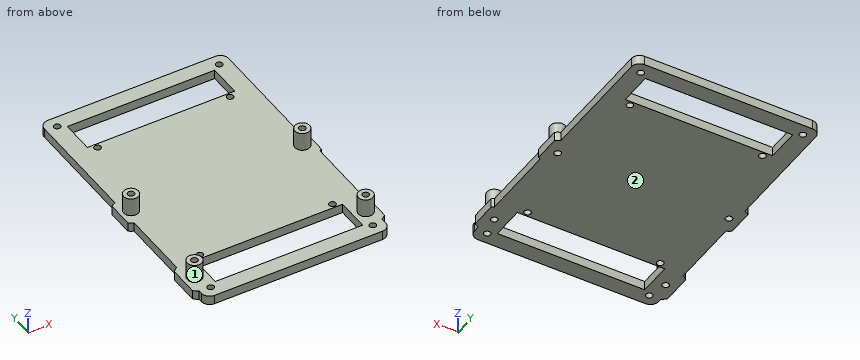
```python
from build123d import *

# Parameters (mm, degrees)
F0_R     = 1.8
F0_W     = 80
F0_H     = 18
F1_DEPTH = 5
F2_R     = 4
F2_R_2   = 1.8
F3_DEPTH = 10


with BuildPart() as f1:
    # F0 (on Top) → F1 (new body)
    with BuildSketch(Plane.XY):
        with BuildLine():
            Line((-50.0234800036, -68.6468068202), (-50.0234800036, -70.5475468516))
            ThreePointArc((-50.0234800036, -70.5475468516), (-48.705460519, -73.7295273669), (-45.5234800036, -75.0475468516))
            Line((-45.5234800036, -75.0475468516), (45.5234800036, -75.0475468516))
            ThreePointArc((45.5234800036, -75.0475468516), (48.705460519, -73.7295273669), (50.0234800036, -70.5475468516))
            Line((50.0234800036, -70.5475468516), (50.0234800036, -67.1066886004))
            ThreePointArc((50.0234800036, -67.1066886004), (51.3336770397, -66.4451599276), (52.5234800036, -65.5857383981))
            Line((52.5234800036, -65.5857383981), (52.5234800036, -51.4142616019))
            ThreePointArc((52.5234800036, -51.4142616019), (51.9046419222, -50.9316550229), (51.2473189859, -50.5029403875))
            Line((51.2473189859, -50.5029403875), (51.2473189859, -9.4970596125))
            ThreePointArc((51.2473189859, -9.4970596125), (51.9046419222, -9.0683449771), (52.5234800036, -8.5857383981))
            Line((52.5234800036, -8.5857383981), (52.5234800036, 5.5857383981))
            ThreePointArc((52.5234800036, 5.5857383981), (51.3336770397, 6.4451599276), (50.0234800036, 7.1066886004))
            Line((50.0234800036, 7.1066886004), (50.0234800036, 70.5475468516))
            ThreePointArc((50.0234800036, 70.5475468516), (48.705460519, 73.7295273669), (45.5234800036, 75.0475468516))
            Line((45.5234800036, 75.0475468516), (-45.5234800036, 75.0475468516))
            ThreePointArc((-45.5234800036, 75.0475468516), (-48.705460519, 73.7295273669), (-50.0234800036, 70.5475468516))
            Line((-50.0234800036, 70.5475468516), (-50.0234800036, 7.1066886004))
            ThreePointArc((-50.0234800036, 7.1066886004), (-51.3336770397, 6.4451599276), (-52.5234800036, 5.5857383981))
            Line((-52.5234800036, 5.5857383981), (-52.5234800036, -8.5857383981))
            ThreePointArc((-52.5234800036, -8.5857383981), (-51.3336770397, -9.4451599276), (-50.0234800036, -10.1066886004))
            Line((-50.0234800036, -10.1066886004), (-50.0234800036, -48.3531931798))
            ThreePointArc((-50.0234800036, -48.3531931798), (-51.3409860595, -49.2614977581), (-52.5234800036, -50.3397127117))
            Line((-52.5234800036, -50.3397127117), (-52.5234800036, -66.6602872883))
            ThreePointArc((-52.5234800036, -66.6602872883), (-51.3409860595, -67.7385022419), (-50.0234800036, -68.6468068202))
        make_face()
        with Locations((-44, -69)):
            Circle(F0_R, mode=Mode.SUBTRACT)
        with Locations((-46.5, -58.5)):
            Circle(F0_R, mode=Mode.SUBTRACT)
        with Locations((-36, -46)):
            Circle(F0_R, mode=Mode.SUBTRACT)
        with Locations((-46.5, -1.5)):
            Circle(F0_R, mode=Mode.SUBTRACT)
        with Locations((0, -57.5)):
            Rectangle(F0_W, F0_H, mode=Mode.SUBTRACT)
        with Locations((44, -69)):
            Circle(F0_R, mode=Mode.SUBTRACT)
        with Locations((46.5, -58.5)):
            Circle(F0_R, mode=Mode.SUBTRACT)
        with Locations((36, -46)):
            Circle(F0_R, mode=Mode.SUBTRACT)
        with Locations((46.5, -1.5)):
            Circle(F0_R, mode=Mode.SUBTRACT)
        with Locations((-36, 46)):
            Circle(F0_R, mode=Mode.SUBTRACT)
        with Locations((-44, 69)):
            Circle(F0_R, mode=Mode.SUBTRACT)
        with Locations((0, 57.5)):
            Rectangle(F0_W, F0_H, mode=Mode.SUBTRACT)
        with Locations((36, 46)):
            Circle(F0_R, mode=Mode.SUBTRACT)
        with Locations((44, 69)):
            Circle(F0_R, mode=Mode.SUBTRACT)
    extrude(amount=F1_DEPTH)

    # F2 (on face) → F3 (join)
    with BuildSketch(Plane.XY.offset(5)):
        with Locations((46.5, -58.5)):
            Circle(F2_R)
        with Locations((46.5, -58.5)):
            Circle(F2_R_2, mode=Mode.SUBTRACT)
        with Locations((-46.5, -58.5)):
            Circle(F2_R)
        with Locations((-46.5, -58.5)):
            Circle(F2_R_2, mode=Mode.SUBTRACT)
        with Locations((-46.5, -1.5)):
            Circle(F2_R)
        with Locations((-46.5, -1.5)):
            Circle(F2_R_2, mode=Mode.SUBTRACT)
        with Locations((46.5, -1.5)):
            Circle(F2_R)
        with Locations((46.5, -1.5)):
            Circle(F2_R_2, mode=Mode.SUBTRACT)
    extrude(amount=F3_DEPTH)


solid = f1.part
```
Check sheet for the modelled part. Datum: model origin and axes. Units: mm. Face numbers are marked on the shaded views. Give positions to 0.01 mm unless a question says otherwise; leave off trailing zeros. Write each loop counter-clockwise with the first axis right and the second up, starting at its lowest first coordinate (ties: lowest second). Pieces come first, ordered by that corner, then holes. Notation, with made-up numbers: (27.25, -34.75) -> (56.25, -34.75) arc R13 ccw to (56.25, -26.75) -> close; hole circle Ø8 at (-36, -39.5). An arc over 180 degrees is marked (long way). Use CSV: the item, a comma, the result in double quotes. Start each with the question number.
Q1. Scan lines: line 1 along X through (y, z) = (-69, 2.6); line 2 along Y through (x, z) = (-26, 0.75); line 3 along Y through (x, z) = (36, 3.9). Record each from-to range of solid material in increasing order.
Q2. Cross-section at A-A on z = 8.5. Enter the section's corners in (x, y).
Q3. Depth check by flat-ended pin: P1, Ø3, axis at x = -40, y = -36, coming from the +Z side; P2, Ø2.5, axis at y = -29, z = 1.5, coming from the -X side; P3, Ø1.5, axis at y = -69, z = 3.5, coming from the -X side. Enter the tip coordinate at first touch or a pass-through.
Q4. Release check for a two-part mould opening along Y. For the marked faces 1 and 2 record: +Y half, -Y half, draft (parallel to the pull), parting line (faces both ways), or undercut.
Q5. Cross-section at C-C on y = 69. Enter the section's corners in (x, z).
Q6. Cross-section at B-B on x = -36. Enter the section's corners in (y, z), and give its area (3 significant figures).
Q7. Cross-section at D-D on x = -25. Enter the section's corners in (y, z).
Working result:
1,line 1,"x = -50.02 to -45.8, -42.2 to 42.2, 45.8 to 50.02"
1,line 2,"y = -75.05 to -66.5, -48.5 to 48.5, 66.5 to 75.05"
1,line 3,"y = -75.05 to -66.5, -48.5 to -47.8, -44.2 to 44.2, 47.8 to 48.5, 66.5 to 75.05"
2,outline,"circle Ø8 at (-46.5, -58.5); circle Ø8 at (-46.5, -1.5); circle Ø8 at (46.5, -58.5); circle Ø8 at (46.5, -1.5); hole circle Ø3.6 at (-46.5, -58.5); hole circle Ø3.6 at (-46.5, -1.5); hole circle Ø3.6 at (46.5, -58.5); hole circle Ø3.6 at (46.5, -1.5)"
3,P1,"stops at z = 5"
3,P2,"stops at x = -50.02"
3,P3,"stops at x = -50.65"
4,face 1,"undercut"
4,face 2,"draft"
5,outline,"(-50.02, 0) -> (-45.8, 0) -> (-45.8, 5) -> (-50.02, 5) -> close; (-42.2, 0) -> (42.2, 0) -> (42.2, 5) -> (-42.2, 5) -> close; (45.8, 0) -> (50.02, 0) -> (50.02, 5) -> (45.8, 5) -> close"
6,outline,"(-75.05, 0) -> (-66.5, 0) -> (-66.5, 5) -> (-75.05, 5) -> close; (-48.5, 0) -> (-47.8, 0) -> (-47.8, 5) -> (-48.5, 5) -> close; (-44.2, 0) -> (44.2, 0) -> (44.2, 5) -> (-44.2, 5) -> close; (47.8, 0) -> (48.5, 0) -> (48.5, 5) -> (47.8, 5) -> close; (66.5, 0) -> (75.05, 0) -> (75.05, 5) -> (66.5, 5) -> close"
6,area,"534 mm^2"
7,outline,"(-75.05, 0) -> (-66.5, 0) -> (-66.5, 5) -> (-75.05, 5) -> close; (-48.5, 0) -> (48.5, 0) -> (48.5, 5) -> (-48.5, 5) -> close; (66.5, 0) -> (75.05, 0) -> (75.05, 5) -> (66.5, 5) -> close"
